```python
from build123d import *

# Parameters (mm, degrees)
F0_W     = 52
F0_H     = 52
F1_DEPTH = 5
F2_W     = 42
F2_H     = 42
F3_DEPTH = 24.5
F4_R     = 1.6
F5_DEPTH = 29.5


# Not quite as in the source:
# - a feature names something its author has since deleted; it is built from what else it names


with BuildPart() as f1:
    # F0 (on Top) → F1 (new body)
    with BuildSketch(Plane.XY):
        Rectangle(F0_W, F0_H)
    extrude(amount=F1_DEPTH)

    # F2 (on face) → F3 (join)
    with BuildSketch(Plane.XY.offset(5)):
        with Locations((0, 5)):
            Rectangle(F2_W, F2_H)
    extrude(amount=F3_DEPTH)

    # F4 (on face) → F5 (cut, through all)
    with BuildSketch(Plane.XY.offset(29.5)):
        with Locations((-15.5, 20.5)):
            Circle(F4_R)
        with Locations((15.5, 20.5)):
            Circle(F4_R)
        with Locations((-15.5, -10.5)):
            Circle(F4_R)
        with Locations((15.5, -10.5)):
            Circle(F4_R)
        with BuildLine():
            ThreePointArc((-11.1, 5), (0, -6.1), (11.1, 5))
            ThreePointArc((11.1, 5), (0, 16.1), (-11.1, 5))
        make_face()
        with BuildLine():
            Line((11.1, -16), (11.1, 5))
            ThreePointArc((11.1, 5), (0, -6.1), (-11.1, 5))
            Line((-11.1, 5), (-11.1, -16))
            Line((-11.1, -16), (11.1, -16))
        make_face()
    extrude(amount=-F5_DEPTH, mode=Mode.SUBTRACT)


solid = f1.part
```
The model under review builds one solid part; all positions refer to its coordinate system, in mm. A direction names the side the tool comes from. Round coordinates to 2 decimals unless told otherwise and drop trailing zeros. Write each loop counter-clockwise with the first axis right and the second up, starting at its lowest first coordinate (ties: lowest second). Pieces come first, ordered by that corner, then holes. Notation, with made-up numbers: (-39, -25.5) -> (-33, -25.5) arc R32 cw to (-33, 11.5) -> close; hole circle Ø4 at (73.25, 34). An arc over 180 degrees is marked (long way). Use CSV: the item, a comma, the result in double quotes.
Q1. For pin 1 Ø6.5 at (y, z) = (-9, 13) entering from +X; pin 2 Ø4 at (y, z) = (-7, 5.5) entering from -X; pin 3 Ø1.5 at (x, z) = (1, 20.5) entering from -Y; pin 4 Ø6 at (y, z) = (-6.5, 25) entering from -X, all flat-tipped, find the tip position at first contact; note any pin that passes through.
Checks:
pin 1,"x = 21"
pin 2,"x = -26"
pin 3,"y = 15.96"
pin 4,"x = -21"
Q2. Mouldability with a two-part tool opening along Y and no side actions: class faces 1 (the flat face through (-16, -16, 17)), 2 (the flat face through (-21, 5, 17)), 3 (the flat face through (0, -16, 3)), 4 (the cylindrical face through (-16.68, 21.58, 14.96)) as released by +Y, released by -Y, zero draft, split by the parting line, or undercut.
Checks:
face 1,"released by -Y"
face 2,"zero draft"
face 3,"undercut"
face 4,"undercut"
Q3. For faces 5 (the flat face through (21, 5, 17)), 6 (the flat face through (0, 19, 29.5)), 7 (the flat face through (0, 26, 15)), 8 (the flat face through (16, -16, 17)), 9 (the flat face through (0, -17, 5)), list the 3-axis set-ups (+Z, -Z, +X, -X, +Y, -Y) from which the entire face can be reached by the end or side of a thin tool; tool diameter is ignored.
Checks:
face 5,"+Z, +X, +Y, -Y"
face 6,"+Z, +X, -X, +Y, -Y"
face 7,"+Z, -Z, +X, -X, +Y"
face 8,"+Z, +X, -X, -Y"
face 9,"+Z, -Y"
Q4. Consider section C-C (x = 0). Give the boundary of the cut face in (y, z).
Checks:
outline,"(-26, 0) -> (-16, 0) -> (-16, 5) -> (-26, 5) -> close; (16.1, 0) -> (26, 0) -> (26, 29.5) -> (16.1, 29.5) -> close"
Q5. Consider section A-A (y = -10.5). Give the boundary of the cut face in (x, z), then the cut area to 3 significant figures.
Checks:
outline,"(-26, 0) -> (-17.1, 0) -> (-17.1, 29.5) -> (-21, 29.5) -> (-21, 5) -> (-26, 5) -> close; (-13.9, 0) -> (-11.1, 0) -> (-11.1, 29.5) -> (-13.9, 29.5) -> close; (11.1, 0) -> (13.9, 0) -> (13.9, 29.5) -> (11.1, 29.5) -> close; (17.1, 0) -> (26, 0) -> (26, 5) -> (21, 5) -> (21, 29.5) -> (17.1, 29.5) -> close"
area,"445 mm²"
Q6. Consider section D-D (z = 14.75). Give the boundary of the cut face in (x, y), then the cut area to 3 significant figures.
Checks:
outline,"(-21, -16) -> (-11.1, -16) -> (-11.1, 5) arc R11.1 cw to (11.1, 5) -> (11.1, -16) -> (21, -16) -> (21, 26) -> (-21, 26) -> close; hole circle Ø3.2 at (-15.5, -10.5); hole circle Ø3.2 at (-15.5, 20.5); hole circle Ø3.2 at (15.5, -10.5); hole circle Ø3.2 at (15.5, 20.5)"
area,"1,070 mm²"
Q7. Consider section B-B (x = -15.5). Give the boundary of the cut face in (y, z), then the cut area to 3 significant figures.
Checks:
outline,"(-26, 0) -> (-12.1, 0) -> (-12.1, 29.5) -> (-16, 29.5) -> (-16, 5) -> (-26, 5) -> close; (-8.9, 0) -> (18.9, 0) -> (18.9, 29.5) -> (-8.9, 29.5) -> close; (22.1, 0) -> (26, 0) -> (26, 29.5) -> (22.1, 29.5) -> close"
area,"1,100 mm²"
Q8. To check wall thickness, follow probe 1 along Y at (x, z) = (-15.5, 8); probe 2 along X at (y, z) = (5.5, 21.75); probe 3 along X at (y, z) = (16.5, 9). State the ranges of each line that lie inside material, in increasing order. Write a range as [from, to].
Checks:
probe 1,"[-16, -12.1], [-8.9, 18.9], [22.1, 26]"
probe 2,"[-21, -11.09], [11.09, 21]"
probe 3,"[-21, 21]"
